Can you work these out from the model? Positions are in its coordinate system, mm. Face numbers are marked on the shaded views. A direction names the side the tool comes from. Round coordinates to 2 decimals unless told otherwise and drop trailing zeros. Loops run counter-clockwise (first coordinate to the right, second up) from the corner with the lowest first, then second, coordinate; pieces in that order, holes last. Notation, with made-up numbers: (-35, 14) -> (-25, 14) arc R22 ccw to (-25, 24) -> close; hole circle Ø11 at (73, -1). An arc over 180 degrees is marked (long way). Use a Markdown table: item, result.
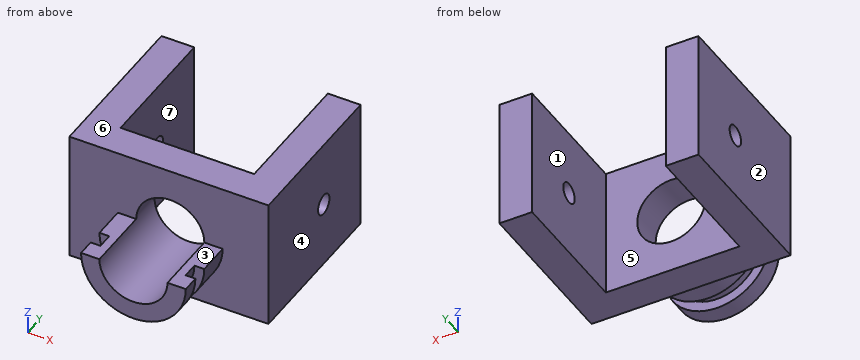
from build123d import *

# Parameters (mm, degrees)
F1_DEPTH  = 20
F2_R      = 5.2
F3_DEPTH  = 25
F5_DEPTH  = 10
F8_DEPTH  = 2.4
F9_R      = 1.55
F10_DEPTH = 40


with BuildPart() as f1:
    # F0 (on Top) → F1 (new body)
    with BuildSketch(Plane.XY):
        Polygon((0, 25), (0, 0), (30.4, 0), (30.4, 25), (25.4, 25), (25.4, 5), (5, 5), (5, 25), align=None)
    extrude(amount=F1_DEPTH)

    # F2 (on face) → F3 (cut)
    with BuildSketch(Plane.XZ):
        with Locations((15.4, 10)):
            Circle(F2_R)
    extrude(amount=-F3_DEPTH, mode=Mode.SUBTRACT)

    # F4 (on face) → F5 (join)
    with BuildSketch(Plane.XZ):
        with BuildLine():
            Line((10.2, 10), (7.4, 10))
            ThreePointArc((7.4, 10), (15.4, 2), (23.4, 10))
            Line((23.4, 10), (20.6, 10))
            ThreePointArc((20.6, 10), (15.4, 4.8), (10.2, 10))
        make_face()
    extrude(amount=F5_DEPTH)

    # F7 (on offset) → F8 (cut)
    with BuildSketch(Plane.XZ.offset(5)):
        with BuildLine():
            Line((23.4, 10), (21.9, 10))
            ThreePointArc((21.9, 10), (15.4, 3.5), (8.9, 10))
            Line((8.9, 10), (7.4, 10))
            ThreePointArc((7.4, 10), (15.4, 2), (23.4, 10))
        make_face()
    extrude(amount=F8_DEPTH, mode=Mode.SUBTRACT)

    # F9 (on face) → F10 (cut)
    with BuildSketch(Plane.YZ.offset(30.4)):
        with Locations((15, 10)):
            Circle(F9_R)
    extrude(amount=-F10_DEPTH, mode=Mode.SUBTRACT)


solid = f1.part
1. Will these pins go through, and if not, where does the flat tip stop? pin 1 Ø1 at (x, z) = (22.5, 14.5) entering from +Y; pin 2 Ø1.4 at (x, y) = (22.5, -7) entering from +Z.
Answer sheet:
| item | result |
|---|---|
| pin 1 | stops at y = 5 |
| pin 2 | stops at z = 10 |
2. I want a section at A-A (y = 15). Please give me the cut outline in (x, z).
Answer sheet:
| item | result |
|---|---|
| outline | (0, 0) -> (5, 0) -> (5, 8.45) -> (0, 8.45) -> close; (0, 11.55) -> (5, 11.55) -> (5, 20) -> (0, 20) -> close; (25.4, 0) -> (30.4, 0) -> (30.4, 8.45) -> (25.4, 8.45) -> close; (25.4, 11.55) -> (30.4, 11.55) -> (30.4, 20) -> (25.4, 20) -> close |
3. I want a section at C-C (z = 5.5). Please give me the cut outline in (x, y), plus the area to 3 significant figures.
Answer sheet:
| item | result |
|---|---|
| outline | (0, 0) -> (8.79, 0) -> (8.79, -5) -> (10.71, -5) -> (10.71, -7.4) -> (8.79, -7.4) -> (8.79, -10) -> (12.79, -10) -> (12.79, 5) -> (5, 5) -> (5, 25) -> (0, 25) -> close; (18.01, -10) -> (22.01, -10) -> (22.01, -7.4) -> (20.09, -7.4) -> (20.09, -5) -> (22.01, -5) -> (22.01, 0) -> (30.4, 0) -> (30.4, 25) -> (25.4, 25) -> (25.4, 5) -> (18.01, 5) -> close |
| area | 397 mm² |
4. I need wall thicknesses on line 1 (X direction, y = 10, z = 10.75); line 2 (Z direction, x = 2, y = 15); line 3 (Y direction, x = 16, z = 1). Which ranges of each line are inside material? Lowest first, please.
Answer sheet:
| item | result |
|---|---|
| line 1 | x = 0 to 5, 25.4 to 30.4 |
| line 2 | z = 0 to 8.45, 11.55 to 20 |
| line 3 | y = 0 to 5 |
5. If we mould it in two halves opening along X, with no side actions, what happens to the marked faces 4, 5, 6 and 7? For each: +X half, -X half, draft (parallel to the pull), parting line (faces both ways), or undercut.
Answer sheet:
| item | result |
|---|---|
| face 4 | +X half |
| face 5 | undercut |
| face 6 | draft |
| face 7 | undercut |
6. Which directions (+Z, -Z, +X, -X, +Y, -Y) give clear straight access to the entire face, cutting with the end or side of a thin tool? Please do the marked faces 1, 2 and 3.
Answer sheet:
| item | result |
|---|---|
| face 1 | +Z, -Z, +Y |
| face 2 | +Z, -Z, -X, +Y, -Y |
| face 3 | +Z, +X, -X, -Y |
7. I want a section at D-D (x = 26.5). Please give me the cut outline in (y, z), plus the area to 3 significant figures.
Answer sheet:
| item | result |
|---|---|
| outline | (0, 0) -> (25, 0) -> (25, 20) -> (0, 20) -> close; hole circle Ø3.1 at (15, 10) |
| area | 492 mm² |
8. I want a section at B-B (x = 15.4). Please give me the cut outline in (y, z), plus the area to 3 significant figures.
Answer sheet:
| item | result |
|---|---|
| outline | (-10, 2) -> (-7.4, 2) -> (-7.4, 3.5) -> (-5, 3.5) -> (-5, 2) -> (0, 2) -> (0, 0) -> (5, 0) -> (5, 4.8) -> (-10, 4.8) -> close; (0, 15.2) -> (5, 15.2) -> (5, 20) -> (0, 20) -> close |
| area | 72.4 mm² |
